Geometry: see drawing. Coordinates: mm, zero at the bounding-box minimum. A direction names the side the tool comes from. Round coordinates to 2 decimals unless told otherwise and drop trailing zeros. Loops run counter-clockwise (first coordinate to the right, second up) from the corner with the lowest first, then second, coordinate; pieces in that order, holes last. Notation, with made-up numbers: (-34.5, 12) - (-20.5, 12) arc R11 cw to (-20.5, 33) - close; hole circle Ø8 at (75.5, 41.25). An arc over 180 degrees is marked (long way). Return JSON: item names as keys, results as strings. Group by question number.
1. Section A-A on x = 15. Return loops of the section in (y, z), and give its area (4 significant figures).
2. Section C-C on z = 62. Return loops of the section in (x, y).
3. Section B-B on y = 21.5. Return loops of the section in (x, z).
4. Set-up query: the marked faces 1, 2, 3, 4 and 5. Return all of +Z, -Z, +X, -X, +Y, -Y with unobstructed straight access to the full face (end or side cutting, diameter ignored); none if empty.
5. Material intervals for probe 1 along X at (y, z) = (10, 45.5); probe 2 along Z at (x, y) = (4.75, 18.5); probe 3 along Z at (x, y) = (28.5, 26.5), sorted ascending.
6. First-contact query: pin 1 Ø12 at (y, z) = (16.5, 32.5) entering from -X; pin 2 Ø3 at (x, z) = (10.5, 47) entering from -Y; pin 3 Ø6 at (x, y) = (7, 16) entering from -Z; pin 4 Ø12 at (x, z) = (6.5, 34.5) entering from +Y. Flat tips, straight axial feed; report the tip coordinate or a pass-through.
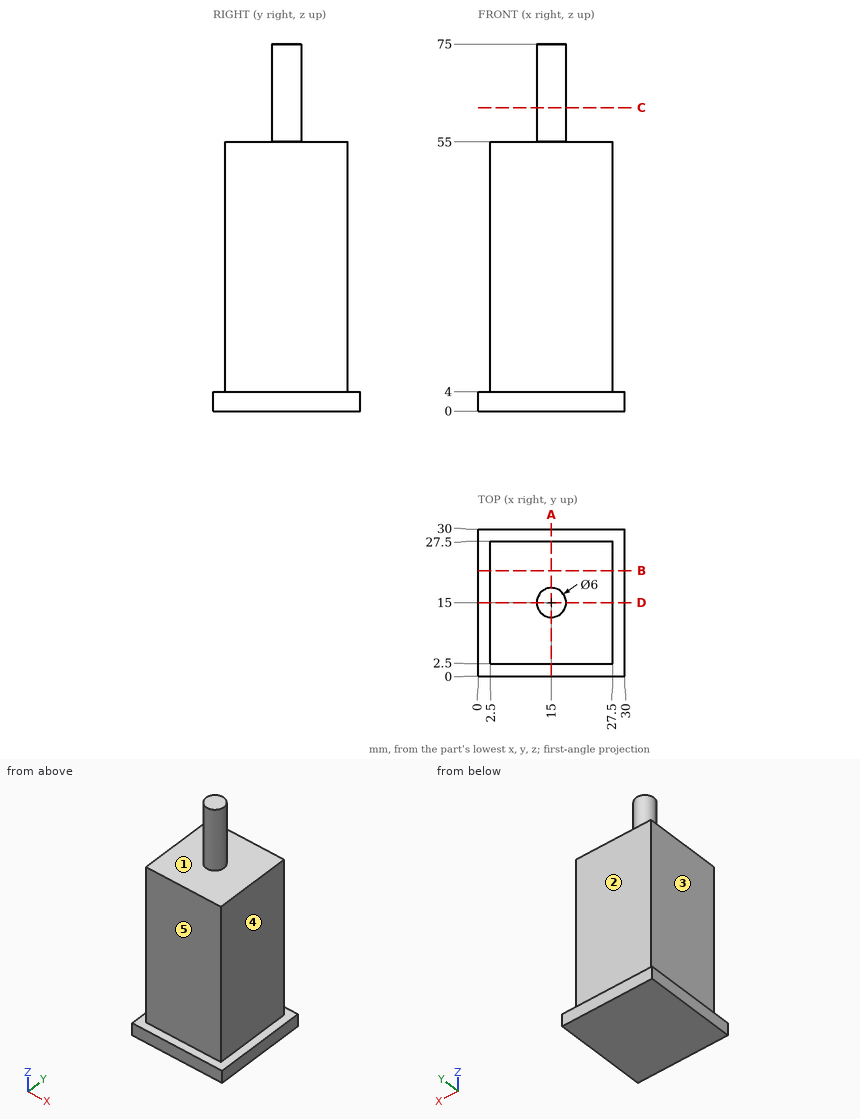
Taken from the geometry:
{
 "1": {"outline": "(0, 0) - (30, 0) - (30, 4) - (27.5, 4) - (27.5, 55) - (18, 55) - (18, 75) - (12, 75) - (12, 55) - (2.5, 55) - (2.5, 4) - (0, 4) - close", "area": "1,515 mm2"},
 "2": {"outline": "circle Ø6 at (15, 15)"},
 "3": {"outline": "(0, 0) - (30, 0) - (30, 4) - (27.5, 4) - (27.5, 55) - (2.5, 55) - (2.5, 4) - (0, 4) - close"},
 "4": {"face 1": "+Z", "face 2": "+Z, +X, -X, +Y", "face 3": "+Z, -X, +Y, -Y", "face 4": "+Z, +X, +Y, -Y", "face 5": "+Z, +X, -X, -Y"},
 "5": {"probe 1": "2.5 to 27.5", "probe 2": "0 to 55", "probe 3": "0 to 4"},
 "6": {"pin 1": "x = 2.5", "pin 2": "y = 2.5", "pin 3": "z = 0", "pin 4": "y = 27.5"}
}
